Design review of the part built by this model. Coordinates are the model's own, in mm. Coordinates: 2 decimals unless noted, no trailing zeros. Loops run counter-clockwise (first coordinate to the right, second up) from the corner with the lowest first, then second, coordinate; pieces in that order, holes last. Notation, with made-up numbers: (11, -13) -> (57, -13) arc R13 ccw to (57, 11) -> close; hole circle Ø6 at (30.25, -5). An arc over 180 degrees is marked (long way). One line per item, written item: value. Start each with the question number.
1. Add section C-C on y = -6.75. Write out the cut boundary in (x, z).
2. Insertion check: pin 1 (2 mm diameter, centred on x = 14, z = 2, fed in from -Y). The pin has a flat end and moves straight along its axis. Give the tip position at first contact, or say it passes through.
3. Draft analysis for pull direction X (two halves, no side actions). For faces 1 (the cylindrical face through (1.44, -1.55, 3.04)), 2 (the flat face through (23, 5.913, 3)), 3 (the flat face through (22.4, -9.5, 2.96)), state which applies: pulls with the +X half, pulls with the -X half, needs draft (parallel to the pull), parting line crosses it, or undercut.
4. Add section A-A on z = 3.25. Write out the cut boundary in (x, y), plus the area to 3 significant figures.
5. For probe 1 along X at (y, z) = (0, 4.5); probe 2 along X at (y, z) = (-0.5, 2.75); probe 3 along Y at (x, z) = (17.5, 4), list the stretches that pass through material, from the lowest coordinate up.
6. Add section D-D on z = 1. Write out the cut boundary in (x, y), plus the area to 3 significant figures.
```python
from build123d import *

# Parameters (mm, degrees)
F1_DEPTH = 6
F2_SIZE  = 5.99999
F3_R     = 1.5
F4_DEPTH = 6


# Not quite as in the source:
# - a fillet or chamfer is up to 0.001 mm smaller than in the source, because OpenCascade refuses the exact size


with BuildPart() as f1:
    # F0 (on Top) → F1 (new body)
    with BuildSketch(Plane.XY):
        Polygon((49.2662842423, 5.9127185345), (-3.7337157577, 5.9127185345), (-3.7337157577, -10.0872814655), (49.2662842423, -15.0872814655), align=None)
    extrude(amount=F1_DEPTH)

    # F2 (size 6 in the source; OpenCascade refuses exactly that, so slightly less here)
    f2_edges = [f1.edges().sort_by_distance(p)[0] for p in [
        (22.766284, -12.587281, 0),
    ]]
    chamfer(f2_edges, length=F2_SIZE)

    # F3 (on face) → F4 (cut, through all)
    with BuildSketch(Plane.XY.offset(6)):
        with Locations((1.7662842423, -0.0872814655)):
            Circle(F3_R)
        with Locations((17.7662842423, -0.0872814655)):
            Circle(F3_R)
        with Locations((27.7662842423, -0.0872814655)):
            Circle(F3_R)
        with Locations((43.7662842423, -0.0872814655)):
            Circle(F3_R)
    extrude(amount=-F4_DEPTH, mode=Mode.SUBTRACT)


solid = f1.part
```
Worked answers:
1. outline: (-3.73, 2.68) -> (24.77, 0) -> (49.27, 0) -> (49.27, 6) -> (-3.73, 6) -> close
2. pin 1: stops at y = -8.75
3. face 1: undercut
3. face 2: needs draft
3. face 3: pulls with the -X half
4. outline: (-3.73, -7.33) -> (49.27, -12.33) -> (49.27, 5.91) -> (-3.73, 5.91) -> close; hole circle Ø3 at (1.77, -0.09); hole circle Ø3 at (17.77, -0.09); hole circle Ø3 at (27.77, -0.09); hole circle Ø3 at (43.77, -0.09)
4. area: 806 mm²
5. probe 1: x = -3.73 to 0.27, 3.26 to 16.27, 19.26 to 26.27, 29.26 to 42.27, 45.26 to 49.27
5. probe 2: x = -3.73 to 0.32, 3.21 to 16.32, 19.21 to 26.32, 29.21 to 42.32, 45.21 to 49.27
5. probe 3: y = -10.08 to -1.56, 1.39 to 5.91
6. outline: (-3.73, -5.07) -> (49.27, -10.07) -> (49.27, 5.91) -> (-3.73, 5.91) -> close; hole circle Ø3 at (1.77, -0.09); hole circle Ø3 at (17.77, -0.09); hole circle Ø3 at (27.77, -0.09); hole circle Ø3 at (43.77, -0.09)
6. area: 686 mm²
